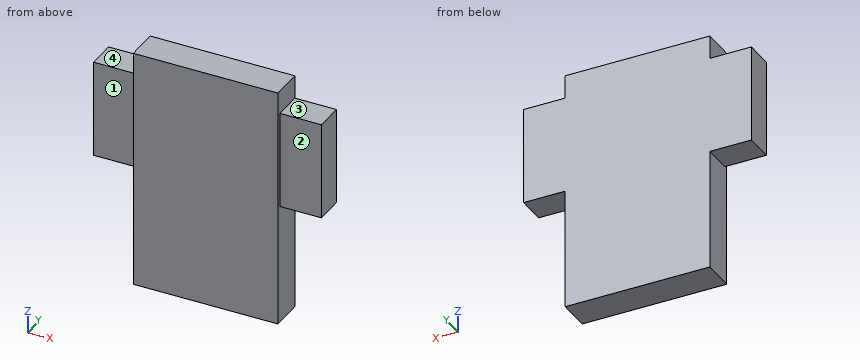
from build123d import *

# Parameters (mm, degrees)
F0_W     = 177.8
F0_H     = 76.2
F1_DEPTH = 22.427941
F2_W     = 112.92833
F2_H     = 189.059824
F3_DEPTH = 25.4


with BuildPart() as f1:
    # F0 (on Front) → F1 (new body)
    with BuildSketch(Plane.XZ):
        Rectangle(F0_W, F0_H)
    extrude(amount=F1_DEPTH)

    # F2 (on Front) → F3 (join)
    with BuildSketch(Plane.XZ):
        with Locations((0, -38.147524)):
            Rectangle(F2_W, F2_H)
    extrude(amount=F3_DEPTH)


solid = f1.part
Geometry: final body of the model. Coordinates: model frame, mm. Face numbers are marked on the shaded views. A direction names the side the tool comes from. Give positions to 0.01 mm unless a question says otherwise; leave off trailing zeros. Loops run counter-clockwise (first coordinate to the right, second up) from the corner with the lowest first, then second, coordinate; pieces in that order, holes last. Notation, with made-up numbers: (65.5, 38) - (112.5, 38) arc R25 ccw to (112.5, 57) - close; hole circle Ø6 at (-21.5, 21). An arc over 180 degrees is marked (long way). Answer as CSV lines item,"result". Start each with the question number.
1. Reachability of the marked faces 1, 2, 3 and 4 from +Z, -Z, +X, -X, +Y, -Y: full face, straight path, thin tool, end or side. Return the list, or none.
2. Section A-A, the plane y = -18.5. Return loops of the section in (x, z), plus the area to 3 significant figures.
3. Section B-B, the plane z = -29.5. Return loops of the section in (x, y).
4. Section C-C, the plane x = -71.5. Return loops of the section in (y, z).
5. Section D-D, the plane z = -75.5. Return loops of the section in (x, y), plus the area to 3 significant figures.
6. Pin query (flat end, axial travel): P1, Ø9.5, axis at x = -79, z = -9.5, coming from the -Y side; P2, Ø4, axis at y = -7.5, z = -61, coming from the +X side; P3, Ø11, axis at x = 80, y = -6.5, coming from the +Z side; P4, Ø10, axis at x = 26, z = -16.5, coming from the +Y side. Return the tip coordinate at first contact, or that it passes through.
7. Ray query, L1, parallel to Z at x = 73.5, y = -19.25; L2, parallel to X at y = -12.75, z = -77; L3, parallel to Y at x = 75, z = -31. Return the intervals inside material, ascending.
Answers:
1,face 1,"+Z, -Z, -X, -Y"
1,face 2,"+Z, -Z, +X, -Y"
1,face 3,"+Z, +X, +Y, -Y"
1,face 4,"+Z, -X, +Y, -Y"
2,outline,"(-88.9, -38.1) - (-56.46, -38.1) - (-56.46, -132.68) - (56.46, -132.68) - (56.46, -38.1) - (88.9, -38.1) - (88.9, 38.1) - (56.46, 38.1) - (56.46, 56.38) - (-56.46, 56.38) - (-56.46, 38.1) - (-88.9, 38.1) - close"
2,area,"26,300 mm2"
3,outline,"(-88.9, -22.43) - (-56.46, -22.43) - (-56.46, -25.4) - (56.46, -25.4) - (56.46, -22.43) - (88.9, -22.43) - (88.9, 0) - (-88.9, 0) - close"
4,outline,"(-22.43, -38.1) - (0, -38.1) - (0, 38.1) - (-22.43, 38.1) - close"
5,outline,"(-56.46, -25.4) - (56.46, -25.4) - (56.46, 0) - (-56.46, 0) - close"
5,area,"2,870 mm2"
6,P1,"stops at y = -22.43"
6,P2,"stops at x = 56.46"
6,P3,"stops at z = 38.1"
6,P4,"stops at y = 0"
7,L1,"z = -38.1 to 38.1"
7,L2,"x = -56.46 to 56.46"
7,L3,"y = -22.43 to 0"
